Read the model definition and answer for the solid it produces. Units are mm, in the model's axes. Face numbers are marked on the shaded views. Round coordinates to 2 decimals unless told otherwise and drop trailing zeros. Order: outer loops, then holes, each group sorted by start corner. A loop starts at its lowest first (then second) coordinate and runs counter-clockwise, first axis right, second up. Notation, with made-up numbers: (48.25, -12.75) -> (55.25, -12.75) arc R33 cw to (55.25, 23.25) -> close; hole circle Ø1 at (80, -12). An arc over 180 degrees is marked (long way). One line per item, written item: value. Start each with the question number.
1. Consider line 1 (Y direction, x = -41, z = 3.25) (3 decimals); line 2 (X direction, y = 20.5, z = 6.5) (3 decimals); line 3 (Z direction, x = -35, y = 5). Determine where each line is inside the solid, lowest interval first.
2. Section C-C (y = -2.5) is taken. Give the vertices of the cut face in (x, z) (3 decimals), then the cut area to 3 significant figures.
3. Section B-B (z = 4.5) is taken. Give the vertices of the cut face in (x, y) (3 decimals), then the cut area to 4 significant figures.
4. Section A-A (x = 20.5) is taken. Give the vertices of the cut face in (y, z) (3 decimals).
5. Flat-ended cylindrical pins translate along their axes: pin 1 Ø2.5 at (x, z) = (-13, 4) entering from -Y (3 decimals); pin 2 Ø1.5 at (y, z) = (5, 4) entering from -X (3 decimals); pin 3 Ø3 at (x, y) = (-15, 24) entering from -Z; pin 4 Ø2.5 at (x, z) = (16, 3.5) entering from +Y (3 decimals). Find the tip coordinate at first contact, or state that the pin passes through.
6. The mould has two halves that part along X. Classify the marked faces 1 and 2: released by +X, released by -X, zero draft, split by the parting line, or undercut.
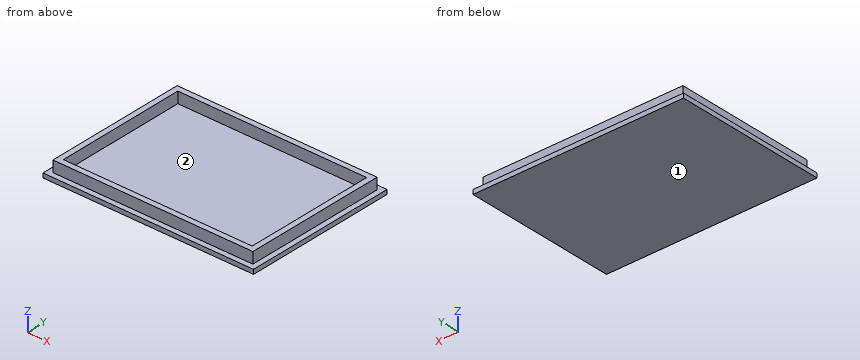
from build123d import *

# Parameters (mm, degrees)
SKETCH_W      = 94.5
SKETCH_H      = 68.5
PAD_DEPTH     = 2
SKETCH001_W   = 89.75
SKETCH001_H   = 63.75
SKETCH001_W_2 = 84.75
SKETCH001_H_2 = 58.75
PAD001_DEPTH  = 5


with BuildPart() as part:
    # Sketch → Pad (new body)
    with BuildSketch(Plane.XY):
        Rectangle(SKETCH_W, SKETCH_H)
    extrude(amount=PAD_DEPTH)

    # Sketch001 (on Face6 of Pad) → Pad001 (join)
    with BuildSketch(Plane.XY.offset(2)):
        Rectangle(SKETCH001_W, SKETCH001_H)
        Rectangle(SKETCH001_W_2, SKETCH001_H_2, mode=Mode.SUBTRACT)
    extrude(amount=PAD001_DEPTH)


solid = part.part
Answer:
1. line 1: -31.875 to -29.375, 29.375 to 31.875
1. line 2: -44.875 to -42.375, 42.375 to 44.875
1. line 3: 0 to 2
2. outline: (-47.25, 0) -> (47.25, 0) -> (47.25, 2) -> (44.875, 2) -> (44.875, 7) -> (42.375, 7) -> (42.375, 2) -> (-42.375, 2) -> (-42.375, 7) -> (-44.875, 7) -> (-44.875, 2) -> (-47.25, 2) -> close
2. area: 214 mm^2
3. outline: (-44.875, -31.875) -> (44.875, -31.875) -> (44.875, 31.875) -> (-44.875, 31.875) -> close; hole (-42.375, -29.375) -> (42.375, -29.375) -> (42.375, 29.375) -> (-42.375, 29.375) -> close
3. area: 742.5 mm^2
4. outline: (-34.25, 0) -> (34.25, 0) -> (34.25, 2) -> (31.875, 2) -> (31.875, 7) -> (29.375, 7) -> (29.375, 2) -> (-29.375, 2) -> (-29.375, 7) -> (-31.875, 7) -> (-31.875, 2) -> (-34.25, 2) -> close
5. pin 1: y = -31.875
5. pin 2: x = -44.875
5. pin 3: z = 0
5. pin 4: y = 31.875
6. face 1: zero draft
6. face 2: undercut
